Check sheet for the modelled part. Datum: model origin and axes. Units: mm. A direction names the side the tool comes from. Round coordinates to 2 decimals unless told otherwise and drop trailing zeros. Loops run counter-clockwise (first coordinate to the right, second up) from the corner with the lowest first, then second, coordinate; pieces in that order, holes last. Notation, with made-up numbers: (78, 76.25) - (90, 76.25) arc R25 cw to (90, 96.25) - close; hole circle Ø8 at (78, -7). An arc over 180 degrees is marked (long way). Answer in a Markdown table with one row per item. Add a question column.
(1) Gauge pin test, flat ends, axial feed: pin 1 (1.5 mm diameter, centred on y = 13.5, z = 0, fed in from +X); pin 2 (2 mm diameter, centred on x = 1, y = 8.5, fed in from +Z); pin 3 (1 mm diameter, centred on x = -1.5, y = 13.5, fed in from +Z). Record the tip position at first contact, or that the pin passes through.
(2) Thickness scan on line 1 along Y through (x, z) = (-1.05, -0.15); line 2 along X through (y, z) = (12, -0.2); line 3 along Y through (x, z) = (-2.2, 0.9). Record the ranges inside material, lowest first.
(3) Cross-section at B-B on y = 8. Enter the section's corners in (x, z), then the cut area to 3 significant figures.
(4) Access from +Z, -Z, +X, -X, +Y, -Y to the whole of each face (thin tool, end or side, straight path). Record for faces 1 (the cylindrical face through (-1.5, 8.04, -0.07)), 2 (the flat face through (0, 0, 0)).
(5) Cross-section at C-C on y = 16.75. Enter the section's corners in (x, z), then the cut area to 3 significant figures.
from build123d import *

# Parameters (mm, degrees)
SKETCH1_R           = 1.5
BOSS_EXTRUDE1_DEPTH = 18
SKETCH2_R           = 2.6
BOSS_EXTRUDE2_DEPTH = 1.7
BOSS_EXTRUDE2_TAPER = 32
SKETCH3_W           = 0.5
SKETCH3_H           = 1.758378485
SKETCH3_H_2         = 1.741621515
SKETCH3_W_2         = 1.734727157
SKETCH3_H_3         = 0.5
SKETCH3_W_3         = 1.765272843
CUT_EXTRUDE1_DEPTH  = 0.3


with BuildPart() as part:
    # Sketch1 → Boss-Extrude1 (new body)
    with BuildSketch(Plane(origin=(0, 0, 0), x_dir=(1, 0, 0), z_dir=(0, 1, 0))):
        Circle(SKETCH1_R)
    extrude(amount=BOSS_EXTRUDE1_DEPTH)

    # Sketch2 → Boss-Extrude2 (add)
    with BuildSketch(Plane(origin=(0, 18, 0), x_dir=(1, 0, 0), z_dir=(0, 1, 0))):
        Circle(SKETCH2_R)
    extrude(amount=-BOSS_EXTRUDE2_DEPTH, taper=BOSS_EXTRUDE2_TAPER)

    # Sketch3 → Cut-Extrude1 (cut)
    with BuildSketch(Plane(origin=(0, 18, 0), x_dir=(1, 0, 0), z_dir=(0, 1, 0))):
        with Locations((-0.015272843, 1.120810757)):
            Rectangle(SKETCH3_W, SKETCH3_H)
        with Locations((-0.015272843, -1.129189243)):
            Rectangle(SKETCH3_W, SKETCH3_H_2)
        with Locations((-1.132636421, -0.008378485)):
            Rectangle(SKETCH3_W_2, SKETCH3_H_3)
        with Locations((1.117363579, -0.008378485)):
            Rectangle(SKETCH3_W_3, SKETCH3_H_3)
        with Locations((-0.015272843, -0.008378485)):
            Rectangle(SKETCH3_W, SKETCH3_H_3)
    extrude(amount=-CUT_EXTRUDE1_DEPTH, mode=Mode.SUBTRACT)


solid = part.part
Answers:
| question | item | result |
|---|---|---|
| 1 | pin 1 | stops at x = 1.5 |
| 1 | pin 2 | stops at z = 1.5 |
| 1 | pin 3 | stops at z = 1.12 |
| 2 | line 1 | y = 0 to 17.7 |
| 2 | line 2 | x = -1.49 to 1.49 |
| 2 | line 3 | y = 17.64 to 18 |
| 3 | outline | circle Ø3 at (0, 0) |
| 3 | area | 7.07 mm^2 |
| 4 | face 1 | -Y |
| 4 | face 2 | +Z, -Z, +X, -X, -Y |
| 5 | outline | circle Ø3.64 at (0, 0) |
| 5 | area | 10.4 mm^2 |
